Read the model definition and answer for the solid it produces. Units are mm, in the model's axes. Round coordinates to 2 decimals unless told otherwise and drop trailing zeros. Order: outer loops, then holes, each group sorted by start corner. A loop starts at its lowest first (then second) coordinate and runs counter-clockwise, first axis right, second up. Notation, with made-up numbers: (-8.75, -39.5) -> (-3.75, -39.5) arc R24 cw to (-3.75, -22.5) -> close; hole circle Ø5 at (81.5, -14.75). An arc over 180 degrees is marked (long way). Answer as a JSON object with one key per item and string values. Group by question number.
Item 1: Consider probe 1 along Y at (x, z) = (13, 1.8); probe 2 along X at (y, z) = (12.5, 0.45); probe 3 along X at (y, z) = (-23.5, 1.8). Determine where each line is inside the solid, lowest interval first. Write a range as from..to.
Item 2: Section C-C, the plane y = 23.5 is taken. Write down the section's boundary in (x, z), plus the area to 3 significant figures.
Item 3: Section B-B, the plane z = 0.95 is taken. Write down the section's boundary in (x, y) (3 decimals).
Item 4: Section D-D, the plane y = 9 is taken. Write down the section's boundary in (x, z).
Item 5: Section A-A, the plane x = 34.5 is taken. Write down the section's boundary in (y, z), plus the area to 3 significant figures.
Autodesk Inventor part; units mm, degrees
ref_plane "YZ Plane" through (0, 0, 0) normal (1, 0, 0) x (0, 1, 0)
ref_plane "XZ Plane" through (0, 0, 0) normal (0, 1, 0) x (-1, 0, 0)
ref_plane "XY Plane" through (0, 0, 0) normal (0, 0, 1) x (1, 0, 0)
sketch "スケッチ1" plane through (0, 0, 0) normal (0, 0, 1) x (1, 0, 0)
  circle A0 centre (0, 0) radius 28.5
  line L0 (0, 28.5) -> (39.5, 28.5)
  line L1 (39.5, 28.5) -> (39.5, -28.5)
  line L2 (39.5, -28.5) -> (0, -28.5)
  line L3 (0, -28.5) -> (0, 28.5)
  point P0 (28.5, 0)
  dimension "d0" = 57
  dimension "d19" = 39.5
extrude "押し出し1" add sketch "スケッチ1" along normal blind 2
sketch "スケッチ3" plane through (0, 0, 2) normal (0, 0, 1) x (1, 0, 0)
  circle A0 centre (0, 0) radius 19
  line L0 (0, 0) -> (13.435, -13.435)
  line L1 (0, 0) -> (19, 0) construction
  line L2 (39.5, 28.5) -> (0, 28.5)
  line L3 (34.5, 28.5) -> (34.5, -28.5)
  line L4 (0, -28.5) -> (39.5, -28.5)
  line L5 (39.5, -28.5) -> (39.5, 28.5)
  point P0 (13.435, 13.435)
  point P1 (-13.435, 13.435)
  point P2 (-13.435, -13.435)
  point P3 (34.5, 23.5)
  point P4 (34.5, -23.5)
  dimension "d22" = 38
  dimension "d23" = 45
  dimension "d26" = 360
  dimension "d28" = 5
  dimension "d29" = 5
  dimension "d37" = 5
hole "穴2" at (13.435, -13.435, 2) at (13.435, 13.435, 2) at (-13.435, 13.435, 2) at (-13.435, -13.435, 2) at (34.5, 23.5, 2) at (34.5, -23.5, 2) direction (0, 0, -1) diameter 3.2 end through all
properties part number "link4_plate2" material "アルミニウム 6061"
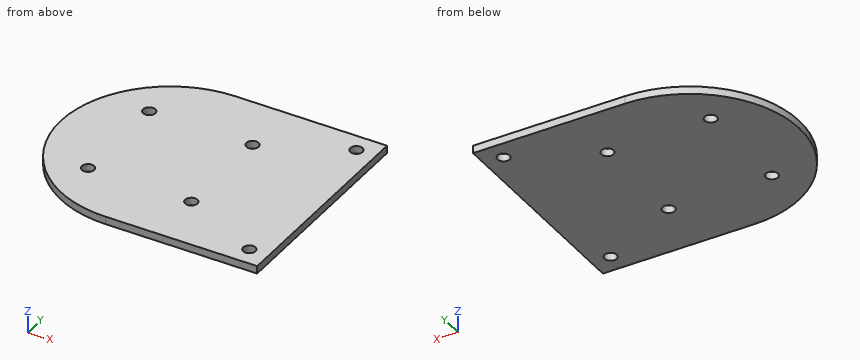
Values found:
{
 "1": {"probe 1": "-28.5..-14.97, -11.9..11.9, 14.97..28.5", "probe 2": "-25.61..-14.73, -12.14..12.14, 14.73..39.5", "probe 3": "-16.12..32.9, 36.1..39.5"},
 "2": {"outline": "(-16.12, 0) -> (32.9, 0) -> (32.9, 2) -> (-16.12, 2) -> close; (36.1, 0) -> (39.5, 0) -> (39.5, 2) -> (36.1, 2) -> close", "area": "105 mm2"},
 "3": {"outline": "(0, -28.5) -> (39.5, -28.5) -> (39.5, 28.5) -> (0, 28.5) arc R28.5 ccw to start; hole circle Ø3.2 at (-13.435, -13.435); hole circle Ø3.2 at (-13.435, 13.435); hole circle Ø3.2 at (13.435, -13.435); hole circle Ø3.2 at (13.435, 13.435); hole circle Ø3.2 at (34.5, -23.5); hole circle Ø3.2 at (34.5, 23.5)"},
 "4": {"outline": "(-27.04, 0) -> (39.5, 0) -> (39.5, 2) -> (-27.04, 2) -> close"},
 "5": {"outline": "(-28.5, 0) -> (-25.1, 0) -> (-25.1, 2) -> (-28.5, 2) -> close; (-21.9, 0) -> (21.9, 0) -> (21.9, 2) -> (-21.9, 2) -> close; (25.1, 0) -> (28.5, 0) -> (28.5, 2) -> (25.1, 2) -> close", "area": "101 mm2"}
}
